from build123d import *

# Parameters (mm, degrees)
SKETCH3_W                                        = 25.4
SKETCH3_H                                        = 7.9375
BOSS_EXTRUDE1_DEPTH                              = 210.5
CSK_FOR_1_4_FLAT_HEAD_MACHINE_SCREW1_D           = 6.7564
CSK_FOR_1_4_FLAT_HEAD_MACHINE_SCREW1_CSINK_D     = 12.8778
CSK_FOR_1_4_FLAT_HEAD_MACHINE_SCREW1_CSINK_ANGLE = 82


with BuildPart() as part:
    # Sketch3 → Boss-Extrude1 (new, symmetric)
    with BuildSketch(Plane.XY):
        Rectangle(SKETCH3_W, SKETCH3_H)
    extrude(amount=BOSS_EXTRUDE1_DEPTH, both=True)

    # CSK for 1/4 Flat Head Machine Screw1 (through all)
    with Locations(Plane(origin=(0, 3.96875, 0), x_dir=(1, 0, 0), z_dir=(0, 1, 0))):
        with Locations((0, 197.8), (0, -197.8), (0, 147), (0, -147)):
            CounterSinkHole(CSK_FOR_1_4_FLAT_HEAD_MACHINE_SCREW1_D / 2, CSK_FOR_1_4_FLAT_HEAD_MACHINE_SCREW1_CSINK_D / 2, counter_sink_angle=CSK_FOR_1_4_FLAT_HEAD_MACHINE_SCREW1_CSINK_ANGLE)


solid = part.part
The listing builds one solid part. Answer for the finished solid, in the listing's coordinates (mm). Round coordinates to 2 decimals unless told otherwise and drop trailing zeros. Write each loop counter-clockwise with the first axis right and the second up, starting at its lowest first coordinate (ties: lowest second). Pieces come first, ordered by that corner, then holes. Notation, with made-up numbers: M -33.75,53.5 L -4.75,53.5 A16 ccw -4.75,58.5 Z; hole C 57,10 d9. An arc over 180 degrees is marked long. Write each question's results on one line, items separated by ' | '. Start each with the question number.
Item 1: Find section A-A on x = 0. Write down the section's boundary in (y, z).
Item 2: The mould has two halves that part along Z. Classify faces 1 (the flat face through (0, 0, 210.5)), 2 (the conical face through (0.765, 0.619, -194.357)), 3 (the flat face through (0, 3.969, 3)): +Z half, -Z half, draft (parallel to the pull), parting line (faces both ways), or undercut.
Item 3: Given pin 1 Ø11 at (x, z) = (0, -147) entering from +Y; pin 2 Ø9 at (x, z) = (0, 197.8) entering from -Y, each flat-ended and moving along its own axis, determine where each tip first touches the part or whether it passes through.
Item 4: Straight lines are drawn through the part: probe 1 along Z at (x, y) = (0, -2.2); probe 2 along X at (y, z) = (-0.85, -197.8); probe 3 along Z at (x, y) = (-1.5, -2). For each, find the intervals that lie inside material, in ascending order.
Item 5: Find section B-B on z = -147. Write down the section's boundary in (x, y), and give its area (3 significant figures).
Answer block:
1) outline: M -3.97,-210.5 L 3.97,-210.5 L 3.97,-204.24 L 0.45,-201.18 L -3.97,-201.18 Z; M -3.97,-194.42 L 0.45,-194.42 L 3.97,-191.36 L 3.97,-153.44 L 0.45,-150.38 L -3.97,-150.38 Z; M -3.97,-143.62 L 0.45,-143.62 L 3.97,-140.56 L 3.97,140.56 L 0.45,143.62 L -3.97,143.62 Z; M -3.97,150.38 L 0.45,150.38 L 3.97,153.44 L 3.97,191.36 L 0.45,194.42 L -3.97,194.42 Z; M -3.97,201.18 L 0.45,201.18 L 3.97,204.24 L 3.97,210.5 L -3.97,210.5 Z
2) face 1: +Z half | face 2: undercut | face 3: draft
3) pin 1: stops at y = 2.89 | pin 2: stops at y = -3.97
4) probe 1: z = -210.5 to -201.18, -194.42 to -150.38, -143.62 to 143.62, 150.38 to 194.42, 201.18 to 210.5 | probe 2: x = -12.7 to -3.38, 3.38 to 12.7 | probe 3: z = -210.5 to -200.83, -194.77 to -150.03, -143.97 to 143.97, 150.03 to 194.77, 200.83 to 210.5
5) outline: M -12.7,-3.97 L -3.38,-3.97 L -3.38,0.45 L -6.44,3.97 L -12.7,3.97 Z; M 3.38,-3.97 L 12.7,-3.97 L 12.7,3.97 L 6.44,3.97 L 3.38,0.45 Z | area: 137 mm²
